Geometry: final body of the model. Coordinates: model frame, mm. A direction names the side the tool comes from. Give positions to 0.01 mm unless a question says otherwise; leave off trailing zeros. Write each loop counter-clockwise with the first axis right and the second up, starting at its lowest first coordinate (ties: lowest second). Pieces come first, ordered by that corner, then holes. Notation, with made-up numbers: (61.5, -10) -> (86.5, -10) arc R32 cw to (86.5, 18) -> close; hole circle Ø3 at (-18.5, 5.5). An arc over 180 degrees is marked (long way). Answer as a JSON object with one key per item and string values.
from build123d import *

# Parameters (mm, degrees)
F0_R     = 24.9809
F1_DEPTH = 279.4
F2_SIZE  = 5.08
F3_R     = 13.942679
F4_DEPTH = 6.35


with BuildPart() as f1:
    # F0 (on Top) → F1 (new body)
    with BuildSketch(Plane.XY):
        Circle(F0_R)
    extrude(amount=F1_DEPTH)

    # F2
    f2_edges = [f1.edges().sort_by_distance(p)[0] for p in [
        (-24.9809, 0, 279.4),
    ]]
    chamfer(f2_edges, length=F2_SIZE)

    # F3 (on face) → F4 (cut)
    with BuildSketch(Plane.XY.offset(279.4)):
        Circle(F3_R)
    extrude(amount=-F4_DEPTH, mode=Mode.SUBTRACT)


solid = f1.part
Q1. Mould query, pull axis Y, two halves, no side actions, for faces 3 (the conical face through (18.611, -7.717, 279.153)), 4 (the flat face through (0, 0, 273.05)), 5 (the flat face through (-14, -4, 279.4)). Classes: pulls with the +Y half, pulls with the -Y half, needs draft (parallel to the pull), parting line crosses it, or undercut.
Values:
{"face 3": "parting line crosses it", "face 4": "undercut", "face 5": "needs draft"}
Q2. First-contact query: P1, Ø10, axis at y = -13.5, z = 52, coming from the -X side; P2, Ø12, axis at x = -11.5, z = 125.5, coming from the -Y side; P3, Ø4, axis at x = 5, z = 247, coming from the +Y side. Flat tips, straight axial feed; report the tip coordinate or a pass-through.
Values:
{"P1": "x = -23.49", "P2": "y = -24.37", "P3": "y = 24.8"}
Q3. Cut plane A-A (z = 155). Return the cut outline in (x, y), and give its area (3 significant figures).
Values:
{"outline": "circle Ø49.96 at (0, 0)", "area": "1,960 mm²"}
Q4. Set-up query: faces 1 (the cylindrical face through (13.3, 4.19, 276.27)), 2 (the cylindrical face through (-3.25, 24.77, 135.24)). Return all of +Z, -Z, +X, -X, +Y, -Y with unobstructed straight access to the full face (end or side cutting, diameter ignored); none if empty.
Values:
{"face 1": "+Z", "face 2": "+Z, -Z"}
Q5. Material intervals for L1, parallel to Y at x = 0, z = 276.25; L2, parallel to Y at x = 0, z = 278; L3, parallel to Z at x = 4, y = -4, sorted ascending. Write a range as from..to.
Values:
{"L1": "-23.05..-13.94, 13.94..23.05", "L2": "-21.3..-13.94, 13.94..21.3", "L3": "0..273.05"}
